Answer from the drawing. Dimensions are ordinates in mm from the lowest x, y and z of the part. Round coordinates to 2 decimals unless told otherwise and drop trailing zeros. Write each loop counter-clockwise with the first axis right and the second up, starting at its lowest first coordinate (ties: lowest second). Pieces come first, ordered by that corner, then holes. Notation, with made-up numbers: (43, -4) - (65, -4) arc R36 ccw to (65, 30) - close; hole circle Ø10 at (-35.5, -14.75). An arc over 180 degrees is marked (long way). Answer in a Markdown table with one row per item.
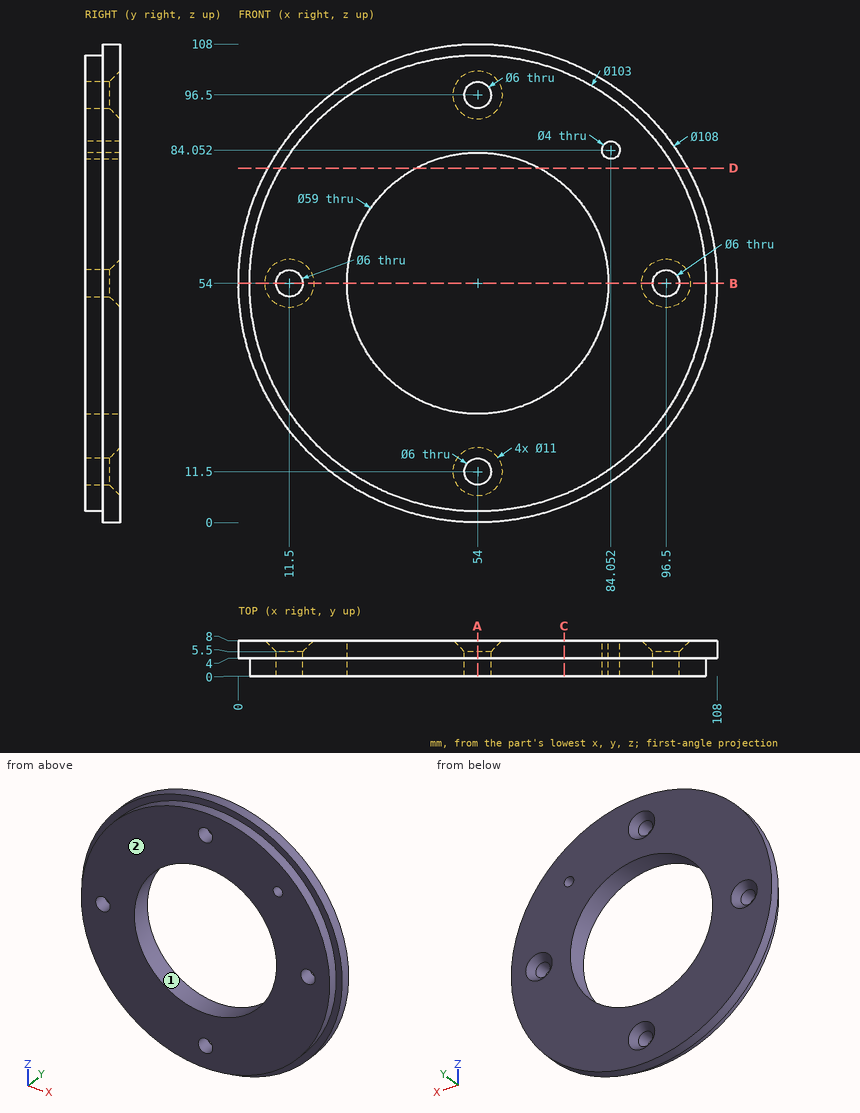
(1) Flat-ended cylindrical pins translate along their axes: pin 1 (9.5 mm diameter, centred on x = 11.5, z = 54, fed in from +Y); pin 2 (1.5 mm diameter, centred on x = 35, y = 2, fed in from -Z); pin 3 (1 mm diameter, centred on y = 5, z = 94, fed in from +X); pin 4 (4.5 mm diameter, centred on x = 84.05, z = 84.05, fed in from -Y). Find the tip coordinate at first contact, or state that the pin passes through.
Checked values:
| item | result |
|---|---|
| pin 1 | stops at y = 7.25 |
| pin 2 | stops at z = 5.84 |
| pin 3 | stops at x = 90.82 |
| pin 4 | stops at y = 0 |
(2) Section D-D (z = 80) is taken. Give the vertices of the cut face in (x, y) (3 decimals), and give its area (3 significant figures).
Checked values:
| item | result |
|---|---|
| outline | (6.671, 4) - (9.545, 4) - (9.545, 0) - (40.063, 0) - (40.063, 8) - (6.671, 8) - close; (67.937, 0) - (98.455, 0) - (98.455, 4) - (101.329, 4) - (101.329, 8) - (67.937, 8) - close |
| area | 511 mm2 |
(3) For a pull along Z with two mould halves and no side action, classify the marked faces 1 and 2 as pulls with the +Z half, pulls with the -Z half, needs draft (parallel to the pull), parting line crosses it, or undercut.
Checked values:
| item | result |
|---|---|
| face 1 | undercut |
| face 2 | needs draft |
(4) Find the intervals of material crossed by line 1 (X direction, y = 2.35, z = 54); line 2 (Z direction, x = 64.5, y = 0.5); line 3 (Z direction, x = 49, y = 6.75), in increasing order.
Checked values:
| item | result |
|---|---|
| line 1 | x = 2.5 to 8.5, 14.5 to 24.5, 83.5 to 93.5, 99.5 to 105.5 |
| line 2 | z = 3.58 to 26.43, 81.57 to 104.42 |
| line 3 | z = 0.23 to 24.93, 83.07 to 107.77 |
(5) Section B-B (z = 54) is taken. Give the vertices of the cut face in (x, y), and give its area (4 significant figures).
Checked values:
| item | result |
|---|---|
| outline | (0, 4) - (2.5, 4) - (2.5, 0) - (8.5, 0) - (8.5, 5.5) - (6, 8) - (0, 8) - close; (14.5, 0) - (24.5, 0) - (24.5, 8) - (17, 8) - (14.5, 5.5) - close; (83.5, 0) - (93.5, 0) - (93.5, 5.5) - (91, 8) - (83.5, 8) - close; (99.5, 0) - (105.5, 0) - (105.5, 4) - (108, 4) - (108, 8) - (102, 8) - (99.5, 5.5) - close |
| area | 263.5 mm2 |
(6) Section A-A (x = 54) is taken. Give the vertices of the cut face in (y, z).
Checked values:
| item | result |
|---|---|
| outline | (0, 2.5) - (4, 2.5) - (4, 0) - (8, 0) - (8, 6) - (5.5, 8.5) - (0, 8.5) - close; (0, 14.5) - (5.5, 14.5) - (8, 17) - (8, 24.5) - (0, 24.5) - close; (0, 83.5) - (8, 83.5) - (8, 91) - (5.5, 93.5) - (0, 93.5) - close; (0, 99.5) - (5.5, 99.5) - (8, 102) - (8, 108) - (4, 108) - (4, 105.5) - (0, 105.5) - close |
(7) Section C-C (x = 73.5) is taken. Give the vertices of the cut face in (y, z), and give its area (3 significant figures).
Checked values:
| item | result |
|---|---|
| outline | (0, 6.33) - (4, 6.33) - (4, 3.64) - (8, 3.64) - (8, 31.86) - (0, 31.86) - close; (0, 76.14) - (8, 76.14) - (8, 104.36) - (4, 104.36) - (4, 101.67) - (0, 101.67) - close |
| area | 430 mm2 |
